from build123d import *

# Parameters (mm, degrees)
SKETCH_W        = 22
SKETCH_H        = 64
PAD_DEPTH       = 9
SKETCH001_W     = 16
SKETCH001_H     = 54.5
POCKET_DEPTH    = 9.001
SKETCH004_W     = 3
SKETCH004_H     = 10
POCKET001_DEPTH = 9.001
SKETCH003_R     = 15
POCKET002_DEPTH = 22.001
SKETCH006_R     = 1.5
POCKET003_DEPTH = 4.75
POCKET004_DEPTH = 2.5
SKETCH007_W     = 1
SKETCH007_H     = 10
PAD001_DEPTH    = 8


with BuildPart() as part:
    # Sketch → Pad (new body)
    with BuildSketch(Plane.XY):
        Rectangle(SKETCH_W, SKETCH_H)
    extrude(amount=PAD_DEPTH)

    # Sketch001 → Pocket (cut, through all)
    with BuildSketch(Plane.XY.offset(9)):
        with Locations((-3, 0)):
            Rectangle(SKETCH001_W, SKETCH001_H)
    extrude(amount=-POCKET_DEPTH, mode=Mode.SUBTRACT)

    # Sketch004 → Pocket001 (cut, through all)
    with BuildSketch(Plane.XY.offset(9)):
        with Locations((6.5, 21.9)):
            Rectangle(SKETCH004_W, SKETCH004_H)
    extrude(amount=-POCKET001_DEPTH, mode=Mode.SUBTRACT)

    # Sketch003 → Pocket002 (cut, through all)
    with BuildSketch(Plane.YZ.offset(11)):
        with Locations((0, -10)):
            Circle(SKETCH003_R)
    extrude(amount=-POCKET002_DEPTH, mode=Mode.SUBTRACT)

    # Sketch006 → Pocket003 (cut)
    with BuildSketch(Plane(origin=(0, 32, 0), x_dir=(-1, 0, 0), z_dir=(0, 1, 0))):
        with Locations((5.5, 4.5)):
            Circle(SKETCH006_R)
    extrude(amount=-POCKET003_DEPTH, mode=Mode.SUBTRACT)

    # Sketch008 → Pocket004 (cut)
    with BuildSketch(Plane.XZ.offset(-27.25)):
        Polygon((-8.45, 6.203183), (-5.5, 7.906367), (-2.55, 6.203183), (-2.55, 2.796817), (-5.5, 1.093633), (-8.45, 2.796817), align=None)
    extrude(amount=-POCKET004_DEPTH, mode=Mode.SUBTRACT)

    # Sketch007 → Pad001 (new body)
    with BuildSketch(Plane(origin=(0, 0, 0), x_dir=(1, 0, 0), z_dir=(0, 0, -1))):
        with Locations((8.5, -21.9)):
            Rectangle(SKETCH007_W, SKETCH007_H)
    extrude(amount=PAD001_DEPTH)


solid = part.part
Design review of the part built by this model. Coordinates are the model's own, in mm. A direction names the side the tool comes from. Round coordinates to 2 decimals unless told otherwise and drop trailing zeros. Order: outer loops, then holes, each group sorted by start corner. A loop starts at its lowest first (then second) coordinate and runs counter-clockwise, first axis right, second up.
1) Consider section D-D (z = -0.75). State the section outline as (x, y) points, plus the area to 3 significant figures.
The answers:
outline: (8, 16.9) - (9, 16.9) - (9, 26.9) - (8, 26.9) - close
area: 10.0 mm2
2) Draft analysis for pull direction Y (two halves, no side actions). For faces 4 (the flat face through (0, 32, 4)), 5 (the flat face through (-11, -30, 4)), 6 (the flat face through (8, 22, 1)), state which applies: released by +Y, released by -Y, zero draft, split by the parting line, or undercut.
The answers:
face 4: released by +Y
face 5: zero draft
face 6: undercut
3) Consider section A-A (x = 0.25). State the section outline as (y, z) points.
The answers:
outline: (-32, 0) - (-27.25, 0) - (-27.25, 9) - (-32, 9) - close; (27.25, 0) - (32, 0) - (32, 9) - (27.25, 9) - close
4) For L1, parallel to Z at x = -5.5, y = 31.5; L2, parallel to Y at x = 0.25, z = 5.75; L3, parallel to X at y = -6.5, z = 5.5, list the stretches that pass through material, from the lowest coordinate up.
The answers:
L1: z = 0 to 3, 6 to 9
L2: y = -32 to -27.25, 27.25 to 32
L3: x = 5 to 11
5) Consider section B-B (z = 1.75). State the section outline as (x, y) points.
The answers:
outline: (-11, -32) - (11, -32) - (11, -9.32) - (5, -9.32) - (5, -27.25) - (-11, -27.25) - close; (-11, 27.25) - (-6.64, 27.25) - (-6.64, 29.75) - (-4.36, 29.75) - (-4.36, 27.25) - (5, 27.25) - (5, 26.9) - (8, 26.9) - (8, 16.9) - (5, 16.9) - (5, 9.32) - (11, 9.32) - (11, 32) - (-11, 32) - close
6) Machinability: for faces 1 (the flat face through (9, 22, -4)), 2 (the flat face through (-3, -27.25, 5)), 3 (the cylindrical face through (-4.3, 30.9, 3.6)), which of the approach directions +Z, -Z, +X, -X, +Y, -Y give a long, thin tool a straight path to every point of the face, cutting with its end or side? Answer none if there is none.
The answers:
face 1: -Z, +X, +Y, -Y
face 2: +Z, -Z, -X
face 3: +Y
7) Consider section C-C (y = 22). State the section outline as (x, z) points, plus the area to 3 significant figures.
The answers:
outline: (8, -8) - (9, -8) - (9, 0) - (11, 0) - (11, 9) - (8, 9) - close
area: 35.0 mm2
8) Clearance check with flat-ended pins moving along their axes: pin 1 Ø0.8 at (x, z) = (8.5, -2.5) entering from -Y; pin 2 Ø1.5 at (y, z) = (5, 7) entering from -X; pin 3 Ø2.5 at (x, z) = (-5.5, 4.5) entering from +Y. State where each tip first meets the part, or that it passes through.
The answers:
pin 1: stops at y = 16.9
pin 2: stops at x = 5
pin 3: stops at y = -27.25
